Could you check a few things on this drawing? It's one solid part, dimensions in mm from its lowest x, y, z. Round coordinates to 2 decimals unless told otherwise and drop trailing zeros. Loops run counter-clockwise (first coordinate to the right, second up) from the corner with the lowest first, then second, coordinate; pieces in that order, holes last. Notation, with made-up numbers: (35.25, 52) -> (48.25, 52) arc R19 ccw to (48.25, 64) -> close; hole circle Ø1 at (39.25, -24). An arc over 180 degrees is marked (long way). Use one line per item in the form item = value. Start each with the question number.
Item 1: If I drill on L1, parallel to Y at x = 70, z = 42; L2, parallel to Z at x = 78, y = 72; L3, parallel to X at y = 53.5, z = 23.5, over which ranges is the centre line in solid material (lowest first)? Write a range as [from, to].
Item 2: If we section it at C-C (z = 44): Write out the boundary of the cut face in (x, y), then the cut area to 3 significant figures.
Item 3: Thinking about a two-plate mould opening in Y: for the marked faces 1, 2 and 3, which applies, released by +Y, released by -Y, zero draft, split by the parting line, or undercut?
Item 4: I'm going to push flat-ended pins straight in: pin 1 Ø3 at (x, y) = (37.5, 92.5) entering from +Z; pin 2 Ø8 at (y, z) = (28, 78.5) entering from +X; pin 3 Ø6 at (x, z) = (93.5, 54.5) entering from +Y. Where does each tip first touch, or does it pass through?
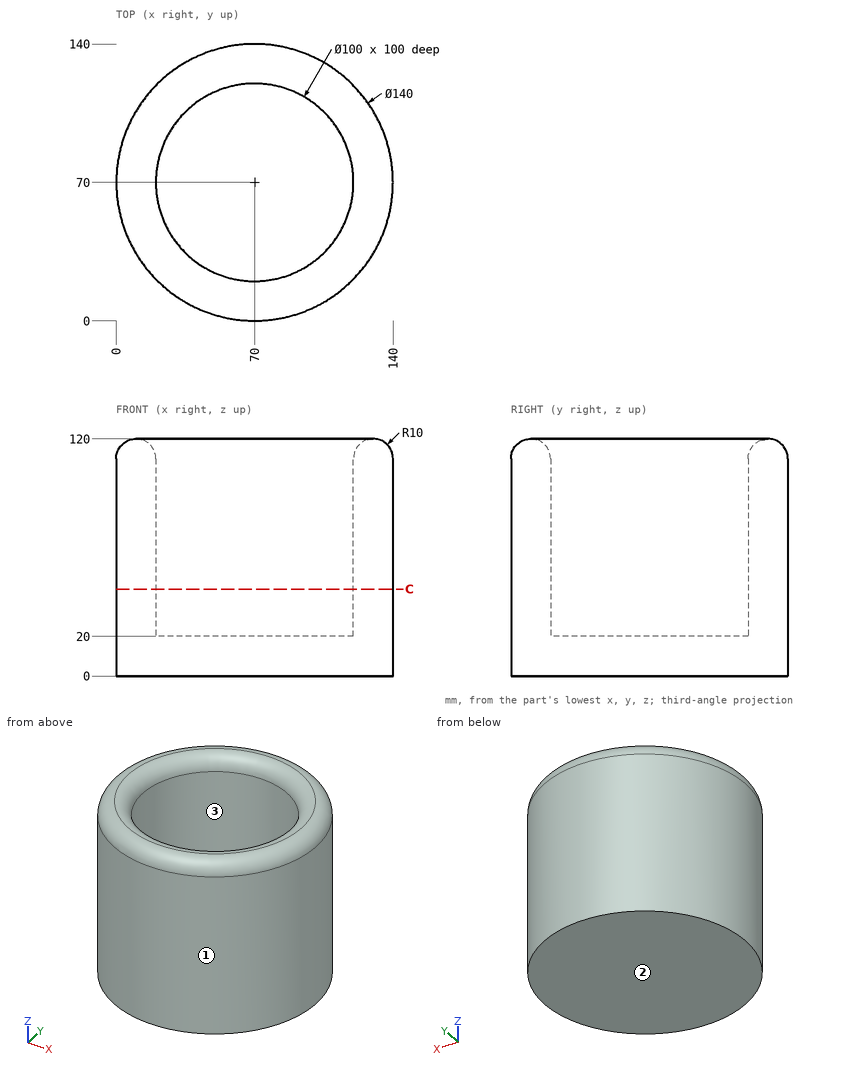
Values found:
q1.L1 = [0, 20], [120, 140]
q1.L2 = [0, 20]
q1.L3 = [1.97, 22.8], [117.2, 138.03]
q2.outline = circle Ø140 at (70, 70); hole circle Ø100 at (70, 70)
q2.area = 7,540 mm2
q3.face_1 = split by the parting line
q3.face_2 = zero draft
q3.face_3 = undercut
q4.pin_1 = 20
q4.pin_2 = 128.79
q4.pin_3 = 136.93
